The listing builds one solid part. Answer for the finished solid, in the listing's coordinates (mm). Give positions to 0.01 mm unless a question says otherwise; leave off trailing zeros. Write each loop counter-clockwise with the first axis right and the second up, starting at its lowest first coordinate (ties: lowest second). Pieces come first, ordered by that corner, then holes. Notation, with made-up numbers: (66.25, 71) - (74.25, 71) arc R17 cw to (74.25, 77) - close; hole circle Ø7 at (64.5, 73.25). An arc over 180 degrees is marked (long way). Write each question's results on one line, items separated by ' | '. Start each with the question number.
Q1. Find the intervals of material crossed by probe 1 along X at (y, z) = (1, -5.25); probe 2 along Z at (x, y) = (23, 13); probe 3 along Y at (x, z) = (-44.5, 1.5), in increasing order.
Q2. Section A-A (y = 40) is taken. Determine the outline of the cut face in (x, z), plus the area to 3 significant figures.
Q3. Flat-ended cylindrical pins translate along their axes: pin 1 Ø1.6 at (x, z) = (39, -3.5) entering from -Y; pin 2 Ø1.8 at (x, z) = (-46.99, -5) entering from -Y; pin 3 Ø5 at (x, z) = (-48.5, -5.5) entering from -Y; pin 4 Ø0.5 at (y, z) = (1, -5) entering from -X. Find the tip coordinate at first contact, or state that the pin passes through.
```python
from build123d import *

# Parameters (mm, degrees)
SALIENTE_EXTRUIR1_DEPTH = 4
CROQUIS2_W              = 10
CROQUIS2_H              = 4
SALIENTE_EXTRUIR2_DEPTH = 10
CROQUIS3_R              = 1.5
CORTAR_EXTRUIR1_DEPTH   = 10
CROQUIS3_3_R            = 1.5
CORTAR_EXTRUIR2_DEPTH   = 1.65
REDONDEO2_R             = 10
CROQUIS4_W              = 4
CROQUIS4_H              = 72
CORTAR_EXTRUIR3_DEPTH   = 4
CORTAR_EXTRUIR4_REACH   = 118.859
CROQUIS5_W              = 80
CROQUIS5_H              = 14.3
REDONDEO3_R             = 3


with BuildPart() as part:
    # Croquis1 → Saliente-Extruir1 (new body)
    with BuildSketch(Plane.XY):
        with BuildLine():
            Line((-98, 60), (-98, -4))
            Line((-98, -4), (90, -4))
            Line((90, -4), (90, 60))
            ThreePointArc((90, 60), (88.94427191, 64.472135955), (86, 68))
            Line((86, 68), (-94, 68))
            ThreePointArc((-94, 68), (-96.94427191, 64.472135955), (-98, 60))
        make_face()
    extrude(amount=SALIENTE_EXTRUIR1_DEPTH)

    # Croquis2 → Saliente-Extruir2 (add)
    with BuildSketch(Plane(origin=(0, 0, 0), x_dir=(-1, 0, 0), z_dir=(0, 0, -1))):
        with Locations((46.991549296, 2)):
            Rectangle(CROQUIS2_W, CROQUIS2_H)
        with Locations((-38.991549296, 2)):
            Rectangle(CROQUIS2_W, CROQUIS2_H)
    extrude(amount=SALIENTE_EXTRUIR2_DEPTH)

    # Croquis3 → Cortar-Extruir1 (cut)
    with BuildSketch(Plane.XZ):
        with Locations((38.991549296, -5)):
            Circle(CROQUIS3_R)
        with Locations((-46.991549296, -5)):
            Circle(CROQUIS3_R)
    extrude(amount=-CORTAR_EXTRUIR1_DEPTH, mode=Mode.SUBTRACT)

    # Croquis3<3> → Cortar-Extruir2 (cut)
    # profile 1 of 2: a face of its own
    with BuildSketch(Plane.XZ):
        Polygon((-46.991549296, -8.175426481), (-44.241549296, -6.58771324), (-44.241549296, -3.41228676), (-46.991549296, -1.824573519), (-49.741549296, -3.41228676), (-49.741549296, -6.58771324), align=None)
        with Locations((-46.991549296, -5)):
            Circle(CROQUIS3_3_R, mode=Mode.SUBTRACT)
    # profile 2 of 2: a face of its own
    with BuildSketch(Plane.XZ):
        Polygon((38.991549296, -8.175426481), (41.741549296, -6.58771324), (41.741549296, -3.41228676), (38.991549296, -1.824573519), (36.241549296, -3.41228676), (36.241549296, -6.58771324), align=None)
        with Locations((38.991549296, -5)):
            Circle(CROQUIS3_3_R, mode=Mode.SUBTRACT)
    extrude(amount=-CORTAR_EXTRUIR2_DEPTH, mode=Mode.SUBTRACT)

    # Redondeo2
    # the kernel refuses this fillet: 10 mm, written as the material it takes off along each edge
    with BuildSketch(Plane(origin=(106, 68, 4), x_dir=(0, -1, 0), z_dir=(-1, 0, 0))) as redondeo2_piece_1:
        with BuildLine():
            CenterArc((8, -10), REDONDEO2_R, 90, 53.130102354)
            Line((0, -4), (-0.16, -3.88))
            ThreePointArc((-0.16, -3.88), (-0.2, -2), (-0.2, 0))
            Line((-0.2, 0), (0, 0.2))
            Line((0, 0.2), (8, 0.2))
            Line((8, 0.2), (8, 0))
        make_face()
    extrude(amount=220, mode=Mode.SUBTRACT)

    # Croquis4 → Cortar-Extruir3 (cut)
    with BuildSketch(Plane.XY.offset(4)):
        with Locations((88, 32)):
            Rectangle(CROQUIS4_W, CROQUIS4_H)
        with Locations((-96, 32)):
            Rectangle(CROQUIS4_W, CROQUIS4_H)
    extrude(amount=-CORTAR_EXTRUIR3_DEPTH, mode=Mode.SUBTRACT)

    # Croquis5 → Cortar-Extruir4 (cut, up to next)
    with BuildSketch(Plane.XY.offset(4), mode=Mode.PRIVATE) as cortar_extruir4_sk1:
        with Locations((-39, 24.95)):
            Rectangle(CROQUIS5_W, CROQUIS5_H)
    cortar_extruir4_tool1 = extrude(cortar_extruir4_sk1.sketch, amount=-CORTAR_EXTRUIR4_REACH, mode=Mode.PRIVATE) & part.part
    add(cortar_extruir4_tool1.solids().sort_by_distance((-39, 24.95, 4))[0], mode=Mode.SUBTRACT)

    # Redondeo3
    redondeo3_edges = [part.edges().sort_by_distance(p)[0] for p in [
        (-79, 17.8, 2),
        (-79, 32.1, 2),
        (1, 32.1, 2),
        (1, 17.8, 2),
    ]]
    fillet(redondeo3_edges, radius=REDONDEO3_R)


solid = part.part
```
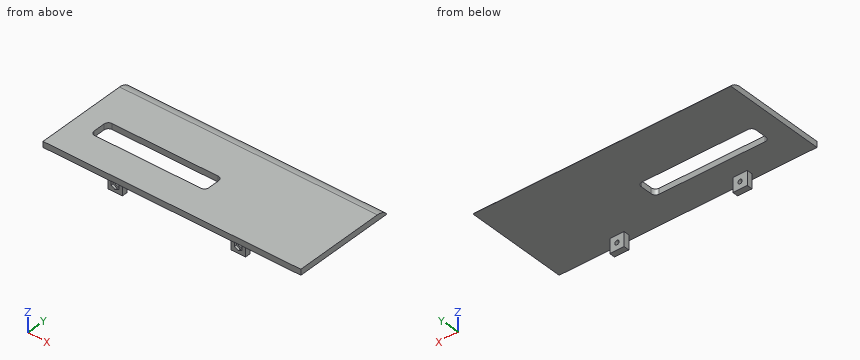
Answers below:
1) probe 1: x = -51.99 to -49.74, -44.24 to -41.99, 33.99 to 36.24, 41.74 to 43.99 | probe 2: z = 0 to 4 | probe 3: y = -4 to 17.8, 32.1 to 66.61
2) outline: (-94, 0) - (86, 0) - (86, 4) - (-94, 4) - close | area: 720 mm2
3) pin 1: stops at y = 1.65 | pin 2: passes through | pin 3: stops at y = 0 | pin 4: stops at x = -51.99
